Geometry check sheet. Reference: the model listing, model coordinates, mm. Give positions to 0.01 mm unless a question says otherwise; leave off trailing zeros. Write each loop counter-clockwise with the first axis right and the second up, starting at its lowest first coordinate (ties: lowest second). Pieces come first, ordered by that corner, then holes.
(1) Cross-section at C-C (y = -2.15). Record the boundary of the cut face in (x, z).
(2) Cross-section at A-A (x = 0). Record the boundary of the cut face in (y, z).
(3) Depth check by flat-ended pin: P1, Ø1.5, axis at y = -2, z = 10.5, coming from the -X side; P2, Ø1.5, axis at x = 14, y = -2.5, coming from the +Z side. Enter the tip coordinate at first touch or a pass-through.
(4) Cross-section at D-D (x = -8). Record the boundary of the cut face in (y, z), and give its area (3 significant figures).
(5) Cross-section at B-B (z = 0). Record the boundary of the cut face in (x, y), and give its area (3 significant figures).
(6) Thickness scan on line 1 along Z through (x, y) = (0, -1); line 2 along X through (y, z) = (-1.15, 1); line 3 along Z through (x, y) = (9, -1.5). Record the ranges inside material, lowest first.
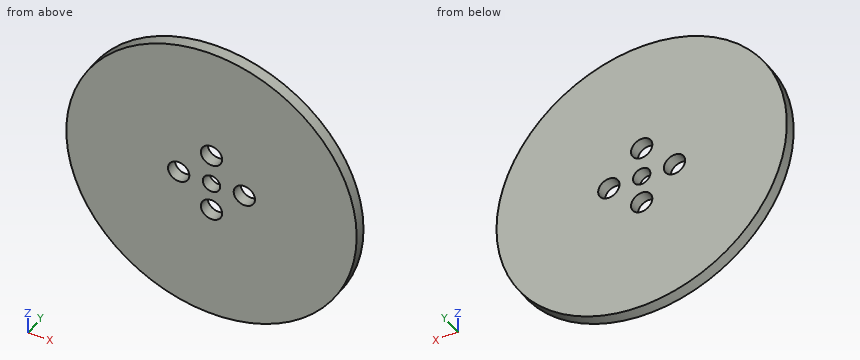
```python
from build123d import *

# Parameters (mm, degrees)
F0_R     = 37.5
F1_DEPTH = 3.048
F2_D     = 4.5
F4_D     = 5.5


with BuildPart() as f1:
    # F0 (on Front) → F1 (new body)
    with BuildSketch(Plane.XZ):
        Circle(F0_R)
    extrude(amount=F1_DEPTH)

    # F2 (through all)
    with Locations(Plane(origin=(0, 0, 0), x_dir=(1, 0, 0), z_dir=(0, 1, 0))):
        with Locations((0, 0)):
            Hole(F2_D / 2)

    # F4 (through all)
    with Locations(Plane(origin=(0, 0, 0), x_dir=(1, 0, 0), z_dir=(0, 1, 0))):
        with Locations((0, -8.0587975681), (-8.4829442203, 0), (0, 7.4932677671), (8.4829442203, 0)):
            Hole(F4_D / 2)


solid = f1.part
```
Reply:
1. outline: circle Ø75 at (0, 0); hole circle Ø5.5 at (-8.48, 0); hole circle Ø5.5 at (0, -7.49); hole circle Ø5.5 at (0, 8.06); hole circle Ø4.5 at (0, 0); hole circle Ø5.5 at (8.48, 0)
2. outline: (-3.05, -37.5) - (0, -37.5) - (0, -10.24) - (-3.05, -10.24) - close; (-3.05, -4.74) - (0, -4.74) - (0, -2.25) - (-3.05, -2.25) - close; (-3.05, 2.25) - (0, 2.25) - (0, 5.31) - (-3.05, 5.31) - close; (-3.05, 10.81) - (0, 10.81) - (0, 37.5) - (-3.05, 37.5) - close
3. P1: stops at x = -36.21
3. P2: stops at z = 35.08
4. outline: (-3.05, -36.64) - (0, -36.64) - (0, -2.71) - (-3.05, -2.71) - close; (-3.05, 2.71) - (0, 2.71) - (0, 36.64) - (-3.05, 36.64) - close
4. area: 207 mm2
5. outline: (-37.5, -3.05) - (-11.23, -3.05) - (-11.23, 0) - (-37.5, 0) - close; (-5.73, -3.05) - (-2.25, -3.05) - (-2.25, 0) - (-5.73, 0) - close; (2.25, -3.05) - (5.73, -3.05) - (5.73, 0) - (2.25, 0) - close; (11.23, -3.05) - (37.5, -3.05) - (37.5, 0) - (11.23, 0) - close
5. area: 181 mm2
6. line 1: z = -37.5 to -10.24, -4.74 to -2.25, 2.25 to 5.31, 10.81 to 37.5
6. line 2: x = -37.49 to -11.04, -5.92 to -2.02, 2.02 to 5.92, 11.04 to 37.49
6. line 3: z = -36.4 to -2.7, 2.7 to 36.4
